from build123d import *

# Parameters (mm, degrees)
CROQUIS1_W              = 80
CROQUIS1_H              = 60
SALIENTE_EXTRUIR1_DEPTH = 40
VACIADO1_T              = -1
CROQUIS2_R              = 2.5
CROQUIS2_R_2            = 1.5
SALIENTE_EXTRUIR2_DEPTH = 40
SALIENTE_EXTRUIR3_DEPTH = 25
CROQUIS4_W              = 1.5
CROQUIS4_H              = 15
CORTAR_EXTRUIR1_DEPTH   = 1
CROQUIS5_R              = 1.5
SALIENTE_EXTRUIR4_DEPTH = 35
CORTAR_EXTRUIR2_REACH   = 82
CROQUIS6_R              = 3.5


with BuildPart() as part:
    # Croquis1 → Saliente-Extruir1 (new body)
    with BuildSketch(Plane.XY):
        Rectangle(CROQUIS1_W, CROQUIS1_H)
    extrude(amount=SALIENTE_EXTRUIR1_DEPTH)

    # Vaciado1
    vaciado1_openings = [part.faces().sort_by_distance(p)[0] for p in [
        (0, 0, 40),
    ]]
    offset(amount=VACIADO1_T, openings=vaciado1_openings, kind=Kind.INTERSECTION)

    # Croquis2 → Saliente-Extruir2 (add)
    with BuildSketch(Plane.XY.offset(40)):
        with Locations((-37.5, 27.5)):
            Circle(CROQUIS2_R)
        with Locations((-37.5, 27.5)):
            Circle(CROQUIS2_R_2, mode=Mode.SUBTRACT)
        with Locations((37.5, 27.5)):
            Circle(CROQUIS2_R)
        with Locations((37.5, 27.5)):
            Circle(CROQUIS2_R_2, mode=Mode.SUBTRACT)
        with Locations((37.5, -27.5)):
            Circle(CROQUIS2_R)
        with Locations((37.5, -27.5)):
            Circle(CROQUIS2_R_2, mode=Mode.SUBTRACT)
        with Locations((-37.5, -27.5)):
            Circle(CROQUIS2_R)
        with Locations((-37.5, -27.5)):
            Circle(CROQUIS2_R_2, mode=Mode.SUBTRACT)
    extrude(amount=-SALIENTE_EXTRUIR2_DEPTH)

    # Croquis3 → Saliente-Extruir3 (add, symmetric)
    with BuildSketch(Plane(origin=(0, 0, 0), x_dir=(0, 0, -1), z_dir=(1, 0, 0))):
        Polygon((-35, -30), (-25.221641576, -39.778358424), (-25.221641576, -37.778358424), (-33.224472237, -29.775527763), (-35, -29.775527763), align=None)
    saliente_extruir3 = extrude(amount=SALIENTE_EXTRUIR3_DEPTH, both=True)

    # Simetría1: Saliente-Extruir3 across plane
    add(saliente_extruir3.mirror(Plane.ZX))

    # Croquis4 → Cortar-Extruir1 (cut)
    with BuildSketch(Plane(origin=(0, 30, 0), x_dir=(1, 0, 0), z_dir=(0, 1, 0))):
        with Locations((5, -25.157633817)):
            Rectangle(CROQUIS4_W, CROQUIS4_H)
        with Locations((0, -25.157633817)):
            Rectangle(CROQUIS4_W, CROQUIS4_H)
        with Locations((10, -25.157633817)):
            Rectangle(CROQUIS4_W, CROQUIS4_H)
        with Locations((15, -25.157633817)):
            Rectangle(CROQUIS4_W, CROQUIS4_H)
        with Locations((20, -25.157633817)):
            Rectangle(CROQUIS4_W, CROQUIS4_H)
        with Locations((-5, -25.157633817)):
            Rectangle(CROQUIS4_W, CROQUIS4_H)
        with Locations((-10, -25.157633817)):
            Rectangle(CROQUIS4_W, CROQUIS4_H)
        with Locations((-15, -25.157633817)):
            Rectangle(CROQUIS4_W, CROQUIS4_H)
        with Locations((-20, -25.157633817)):
            Rectangle(CROQUIS4_W, CROQUIS4_H)
    cortar_extruir1 = extrude(amount=-CORTAR_EXTRUIR1_DEPTH, mode=Mode.SUBTRACT)

    # Simetría2: Cortar-Extruir1 across plane
    add(cortar_extruir1.mirror(Plane.ZX), mode=Mode.SUBTRACT)

    # Croquis5 → Saliente-Extruir4 (add)
    with BuildSketch(Plane.XY.offset(1)):
        with Locations((37.5, -27.5)):
            Circle(CROQUIS5_R)
        with Locations((37.5, 27.5)):
            Circle(CROQUIS5_R)
        with Locations((-37.5, 27.5)):
            Circle(CROQUIS5_R)
        with Locations((-37.5, -27.5)):
            Circle(CROQUIS5_R)
    extrude(amount=SALIENTE_EXTRUIR4_DEPTH)

    # Croquis6 → Cortar-Extruir2 (cut, up to next)
    with BuildSketch(Plane.ZY.offset(40), mode=Mode.PRIVATE) as cortar_extruir2_sk1:
        with Locations((10, -20)):
            Circle(CROQUIS6_R)
    cortar_extruir2_tool1 = extrude(cortar_extruir2_sk1.sketch, amount=-CORTAR_EXTRUIR2_REACH, mode=Mode.PRIVATE) & part.part
    add(cortar_extruir2_tool1.solids().sort_by_distance((-40, -20, 10))[0], mode=Mode.SUBTRACT)


solid = part.part
For this review, take the finished solid that the model builds, in its own axes (mm). A direction names the side the tool comes from. Round coordinates to 2 decimals unless told otherwise and drop trailing zeros. Write each loop counter-clockwise with the first axis right and the second up, starting at its lowest first coordinate (ties: lowest second). Pieces come first, ordered by that corner, then holes. Notation, with made-up numbers: (1.25, 11) -> (40.25, 11) arc R30 cw to (40.25, 43) -> close; hole circle Ø6 at (17.5, 4.25). An arc over 180 degrees is marked (long way). Use CSV: the item, a comma, the result in double quotes.
(1) Consider section A-A, the plane z = 37. Give the boundary of the cut face in (x, y), plus the area to 3 significant figures.
Computed values:
outline,"(-40, -30) -> (40, -30) -> (40, 30) -> (-40, 30) -> close; hole circle Ø3 at (-37.5, -27.5); hole (-39, -25.5) arc R2.5 cw to (-35.5, -29) -> (35.5, -29) arc R2.5 cw to (39, -25.5) -> (39, 25.5) arc R2.5 cw to (35.5, 29) -> (-35.5, 29) arc R2.5 cw to (-39, 25.5) -> close; hole circle Ø3 at (-37.5, 27.5); hole circle Ø3 at (37.5, -27.5); hole circle Ø3 at (37.5, 27.5)"
area,"304 mm²"
(2) Consider section B-B, the plane x = -28. Give the boundary of the cut face in (y, z).
Computed values:
outline,"(-30, 0) -> (30, 0) -> (30, 40) -> (29, 40) -> (29, 1) -> (-29, 1) -> (-29, 40) -> (-30, 40) -> close"
(3) Draft analysis for pull direction Y (two halves, no side actions). For faces 5 (the face through (-25, 34, 30)), 6 (the face through (37, 28, 36)), 7 (the face through (0, 35, 30)), 8 (the face through (35.697, 25.768, 20.773)), state which applies: +Y half, -Y half, draft (parallel to the pull), parting line (faces both ways), or undercut.
Computed values:
face 5,"draft"
face 6,"undercut"
face 7,"+Y half"
face 8,"undercut"
(4) Consider section C-C, the plane z = 4.5. Give the boundary of the cut face in (x, y).
Computed values:
outline,"(-40, -30) -> (40, -30) -> (40, 30) -> (-40, 30) -> close; hole (-39, -25.5) arc R2.5 cw to (-35.5, -29) -> (35.5, -29) arc R2.5 cw to (39, -25.5) -> (39, 25.5) arc R2.5 cw to (35.5, 29) -> (-35.5, 29) arc R2.5 cw to (-39, 25.5) -> close"
(5) To check wall thickness, follow L1, parallel to X at y = 27.5, z = 37.65; L2, parallel to Y at x = 37.5, z = 39.1; L3, parallel to Y at x = 36, z = 35.5. State the ranges of each line that lie inside material, in increasing order. Write a range as [from, to].
Computed values:
L1,"[-40, -39], [-36, -35], [35, 36], [39, 40]"
L2,"[-30, -29], [-26, -25], [25, 26], [29, 30]"
L3,"[-30, -25.5], [25.5, 30]"
(6) Consider section D-D, the plane y = -27.5. Give the boundary of the cut face in (x, z).
Computed values:
outline,"(-40, 0) -> (40, 0) -> (40, 40) -> (39, 40) -> (39, 36) -> (36, 36) -> (36, 40) -> (35, 40) -> (35, 1) -> (-35, 1) -> (-35, 40) -> (-36, 40) -> (-36, 36) -> (-39, 36) -> (-39, 40) -> (-40, 40) -> close"
(7) Clearance check with flat-ended pins moving along their axes: P1, Ø1.5, axis at x = 25.5, z = 23, coming from the -Y side; P2, Ø2, axis at x = 26, z = 19, coming from the +Y side; P3, Ø0.9, axis at x = 38, y = -27, coming from the +Z side. State where each tip first meets the part, or that it passes through.
Computed values:
P1,"y = -30"
P2,"y = 30"
P3,"z = 36"
(8) For faces 1 (the face through (25, -34, 30)), 2 (the face through (0, -29, 16)), 3 (the face through (0, -35, 30)), 4 (the face through (0, -39, 25.222)), list the 3-axis set-ups (+Z, -Z, +X, -X, +Y, -Y) from which the entire face can be reached by the end or side of a thin tool; tool diameter is ignored.
Computed values:
face 1,"+Z, -Z, +X, -Y"
face 2,"+Z"
face 3,"+Z, +X, -X, -Y"
face 4,"-Z, +X, -X, -Y"
